from build123d import *

# Parameters (mm, degrees)
Y_KSEKLIK_EKSTR_ZYON1_DEPTH = 5
Y_KSEKLIK_EKSTR_ZYON2_DEPTH = 11.35
Y_KSEKLIK_EKSTR_ZYON3_DEPTH = 2.45
Y_KSEKLIK_EKSTR_ZYON4_DEPTH = 4
IZIM5_R                     = 5.65
Y_KSEKLIK_EKSTR_ZYON5_DEPTH = 4.3
IZIM7_R                     = 0.75
Y_KSEKLIK_EKSTR_ZYON6_DEPTH = 2.9
RADYUS1_R                   = 0.1
IZIM8_R                     = 0.6
Y_KSEKLIK_EKSTR_ZYON7_DEPTH = 3
SKETCH1_OUTSIDE_W           = 23.446
SKETCH1_OUTSIDE_H           = 43.396
SKETCH1_OUTSIDE_W_2         = 11.9
SKETCH1_OUTSIDE_H_2         = 23.420918094
CUT_EXTRUDE1_DEPTH          = 2.45


with BuildPart() as part:
    # Çizim1 → Yükseklik-Ekstrüzyon1 (new body)
    with BuildSketch(Plane(origin=(0, 0, 0), x_dir=(1, 0, 0), z_dir=(0, 1, 0))):
        with BuildLine():
            Line((-5.65, -11.425), (5.65, -11.425))
            ThreePointArc((5.65, -11.425), (6.003553391, -11.278553391), (6.15, -10.925))
            Line((6.15, -10.925), (6.15, 10.925))
            ThreePointArc((6.15, 10.925), (6.003553391, 11.278553391), (5.65, 11.425))
            Line((5.65, 11.425), (-5.65, 11.425))
            ThreePointArc((-5.65, 11.425), (-6.003553391, 11.278553391), (-6.15, 10.925))
            Line((-6.15, 10.925), (-6.15, -10.925))
            ThreePointArc((-6.15, -10.925), (-6.003553391, -11.278553391), (-5.65, -11.425))
        make_face()
    extrude(amount=Y_KSEKLIK_EKSTR_ZYON1_DEPTH)

    # Çizim2 → Yükseklik-Ekstrüzyon2 (add)
    with BuildSketch(Plane(origin=(0, 5, 0), x_dir=(1, 0, 0), z_dir=(0, 1, 0))):
        with BuildLine():
            Line((-5.6, -11.35), (5.6, -11.35))
            ThreePointArc((5.6, -11.35), (5.953553391, -11.203553391), (6.1, -10.85))
            Line((6.1, -10.85), (6.1, 10.85))
            ThreePointArc((6.1, 10.85), (5.953553391, 11.203553391), (5.6, 11.35))
            Line((5.6, 11.35), (-5.6, 11.35))
            ThreePointArc((-5.6, 11.35), (-5.953553391, 11.203553391), (-6.1, 10.85))
            Line((-6.1, 10.85), (-6.1, -10.85))
            ThreePointArc((-6.1, -10.85), (-5.953553391, -11.203553391), (-5.6, -11.35))
        make_face()
    extrude(amount=Y_KSEKLIK_EKSTR_ZYON2_DEPTH)

    # Çizim3 → Yükseklik-Ekstrüzyon3 (add)
    with BuildSketch(Plane(origin=(0, 16.35, 0), x_dir=(1, 0, 0), z_dir=(0, 1, 0))):
        with BuildLine():
            Line((-5.95, 15.625), (-5.95, 11.207071421))
            ThreePointArc((-5.95, 11.207071421), (-5.789029481, 11.31289076), (-5.6, 11.35))
            Line((-5.6, 11.35), (5.6, 11.35))
            ThreePointArc((5.6, 11.35), (5.789029481, 11.31289076), (5.95, 11.207071421))
            Line((5.95, 11.207071421), (5.95, 15.625))
            ThreePointArc((5.95, 15.625), (5.803553391, 15.978553391), (5.45, 16.125))
            Line((5.45, 16.125), (0.5, 16.125))
            Line((0.5, 16.125), (0.5, 14.991025404))
            ThreePointArc((0.5, 14.991025404), (0, 13.125), (-0.5, 14.991025404))
            Line((-0.5, 14.991025404), (-0.5, 16.125))
            Line((-0.5, 16.125), (-5.45, 16.125))
            ThreePointArc((-5.45, 16.125), (-5.803553391, 15.978553391), (-5.95, 15.625))
        make_face()
        with BuildLine():
            Line((-5.95, 11.207071421), (-5.95, -11.207071421))
            ThreePointArc((-5.95, -11.207071421), (-5.789029481, -11.31289076), (-5.6, -11.35))
            Line((-5.6, -11.35), (5.6, -11.35))
            ThreePointArc((5.6, -11.35), (5.789029481, -11.31289076), (5.95, -11.207071421))
            Line((5.95, -11.207071421), (5.95, 11.207071421))
            ThreePointArc((5.95, 11.207071421), (5.789029481, 11.31289076), (5.6, 11.35))
            Line((5.6, 11.35), (-5.6, 11.35))
            ThreePointArc((-5.6, 11.35), (-5.789029481, 11.31289076), (-5.95, 11.207071421))
        make_face()
        with BuildLine():
            ThreePointArc((-5.95, -15.625), (-5.803553391, -15.978553391), (-5.45, -16.125))
            Line((-5.45, -16.125), (-0.5, -16.125))
            Line((-0.5, -16.125), (-0.5, -14.991025404))
            ThreePointArc((-0.5, -14.991025404), (0, -13.125), (0.5, -14.991025404))
            Line((0.5, -14.991025404), (0.5, -16.125))
            Line((0.5, -16.125), (5.45, -16.125))
            ThreePointArc((5.45, -16.125), (5.803553391, -15.978553391), (5.95, -15.625))
            Line((5.95, -15.625), (5.95, -11.207071421))
            ThreePointArc((5.95, -11.207071421), (5.789029481, -11.31289076), (5.6, -11.35))
            Line((5.6, -11.35), (-5.6, -11.35))
            ThreePointArc((-5.6, -11.35), (-5.789029481, -11.31289076), (-5.95, -11.207071421))
            Line((-5.95, -11.207071421), (-5.95, -15.625))
        make_face()
    extrude(amount=Y_KSEKLIK_EKSTR_ZYON3_DEPTH)

    # Çizim4 → Yükseklik-Ekstrüzyon4 (add)
    with BuildSketch(Plane(origin=(0, 18.8, 0), x_dir=(1, 0, 0), z_dir=(0, 1, 0))):
        with BuildLine():
            Line((-5.4, -11.2), (5.4, -11.2))
            ThreePointArc((5.4, -11.2), (5.753553391, -11.053553391), (5.9, -10.7))
            Line((5.9, -10.7), (5.9, 10.7))
            ThreePointArc((5.9, 10.7), (5.753553391, 11.053553391), (5.4, 11.2))
            Line((5.4, 11.2), (-5.4, 11.2))
            ThreePointArc((-5.4, 11.2), (-5.753553391, 11.053553391), (-5.9, 10.7))
            Line((-5.9, 10.7), (-5.9, -10.7))
            ThreePointArc((-5.9, -10.7), (-5.753553391, -11.053553391), (-5.4, -11.2))
        make_face()
    extrude(amount=Y_KSEKLIK_EKSTR_ZYON4_DEPTH)

    # Çizim5 → Yükseklik-Ekstrüzyon5 (add)
    with BuildSketch(Plane(origin=(0, 22.8, 0), x_dir=(1, 0, 0), z_dir=(0, 1, 0))):
        with Locations((0, 5.45)):
            Circle(IZIM5_R)
        with BuildLine():
            ThreePointArc((-2.6, -0.85), (0, -3.45), (2.6, -0.85))
            Line((2.6, -0.85), (2.6, 0.433776321))
            ThreePointArc((2.6, 0.433776321), (0, -0.2), (-2.6, 0.433776321))
            Line((-2.6, 0.433776321), (-2.6, -0.85))
        make_face()
    extrude(amount=Y_KSEKLIK_EKSTR_ZYON5_DEPTH)

    # Çizim7 → Yükseklik-Ekstrüzyon6 (add)
    # profile 1 of 21: a face of its own
    with BuildSketch(Plane(origin=(0, 27.1, 0), x_dir=(1, 0, 0), z_dir=(0, 1, 0))):
        Polygon((1.982489516, 6.460128862), (1.573312588, 7.023312588), (1.010128862, 7.432489516), (0.348066685, 7.647606558), (-0.348066685, 7.647606558), (-1.010128862, 7.432489516), (-1.573312588, 7.023312588), (-1.982489516, 6.460128862), (-2.197606558, 5.798066685), (-2.197606558, 5.101933315), (-1.982489516, 4.439871138), (-1.573312588, 3.876687412), (-1.010128862, 3.467510484), (-0.348066685, 3.252393442), (0.348066685, 3.252393442), (1.010128862, 3.467510484), (1.573312588, 3.876687412), (1.982489516, 4.439871138), (2.197606558, 5.101933315), (2.197606558, 5.798066685), align=None)
        with Locations(Location((0, 5.45, 0), (0, 0, 270))):
            Circle(IZIM7_R, mode=Mode.SUBTRACT)
    # profile 2 of 21: a face of its own
    with BuildSketch(Plane(origin=(0, 27.1, 0), x_dir=(1, 0, 0), z_dir=(0, 1, 0))):
        Polygon((-0.749366211, 7.756312052), (-0.348066685, 7.647606558), (-1.010128862, 7.432489516), align=None)
    # profile 3 of 21: a face of its own
    with BuildSketch(Plane(origin=(0, 27.1, 0), x_dir=(1, 0, 0), z_dir=(0, 1, 0))):
        Polygon((0, 7.875), (0.348066685, 7.647606558), (-0.348066685, 7.647606558), align=None)
    # profile 4 of 21: a face of its own
    with BuildSketch(Plane(origin=(0, 27.1, 0), x_dir=(1, 0, 0), z_dir=(0, 1, 0))):
        Polygon((-1.425379237, 7.411866211), (-1.010128862, 7.432489516), (-1.573312588, 7.023312588), align=None)
    # profile 5 of 21: a face of its own
    with BuildSketch(Plane(origin=(0, 27.1, 0), x_dir=(1, 0, 0), z_dir=(0, 1, 0))):
        Polygon((-1.961866211, 6.875379237), (-1.573312588, 7.023312588), (-1.982489516, 6.460128862), align=None)
    # profile 6 of 21: a face of its own
    with BuildSketch(Plane(origin=(0, 27.1, 0), x_dir=(1, 0, 0), z_dir=(0, 1, 0))):
        Polygon((-2.306312052, 6.199366211), (-1.982489516, 6.460128862), (-2.197606558, 5.798066685), align=None)
    # profile 7 of 21: a face of its own
    with BuildSketch(Plane(origin=(0, 27.1, 0), x_dir=(1, 0, 0), z_dir=(0, 1, 0))):
        Polygon((-2.306312052, 4.700633789), (-2.197606558, 5.101933315), (-1.982489516, 4.439871138), align=None)
    # profile 8 of 21: a face of its own
    with BuildSketch(Plane(origin=(0, 27.1, 0), x_dir=(1, 0, 0), z_dir=(0, 1, 0))):
        Polygon((-2.425, 5.45), (-2.197606558, 5.798066685), (-2.197606558, 5.101933315), align=None)
    # profile 9 of 21: a face of its own
    with BuildSketch(Plane(origin=(0, 27.1, 0), x_dir=(1, 0, 0), z_dir=(0, 1, 0))):
        Polygon((-1.961866211, 4.024620763), (-1.982489516, 4.439871138), (-1.573312588, 3.876687412), align=None)
    # profile 10 of 21: a face of its own
    with BuildSketch(Plane(origin=(0, 27.1, 0), x_dir=(1, 0, 0), z_dir=(0, 1, 0))):
        Polygon((-1.425379237, 3.488133789), (-1.573312588, 3.876687412), (-1.010128862, 3.467510484), align=None)
    # profile 11 of 21: a face of its own
    with BuildSketch(Plane(origin=(0, 27.1, 0), x_dir=(1, 0, 0), z_dir=(0, 1, 0))):
        Polygon((-0.749366211, 3.143687948), (-1.010128862, 3.467510484), (-0.348066685, 3.252393442), align=None)
    # profile 12 of 21: a face of its own
    with BuildSketch(Plane(origin=(0, 27.1, 0), x_dir=(1, 0, 0), z_dir=(0, 1, 0))):
        Polygon((0, 3.025), (-0.348066685, 3.252393442), (0.348066685, 3.252393442), align=None)
    # profile 13 of 21: a face of its own
    with BuildSketch(Plane(origin=(0, 27.1, 0), x_dir=(1, 0, 0), z_dir=(0, 1, 0))):
        Polygon((0.749366211, 3.143687948), (0.348066685, 3.252393442), (1.010128862, 3.467510484), align=None)
    # profile 14 of 21: a face of its own
    with BuildSketch(Plane(origin=(0, 27.1, 0), x_dir=(1, 0, 0), z_dir=(0, 1, 0))):
        Polygon((0.749366211, 7.756312052), (1.010128862, 7.432489516), (0.348066685, 7.647606558), align=None)
    # profile 15 of 21: a face of its own
    with BuildSketch(Plane(origin=(0, 27.1, 0), x_dir=(1, 0, 0), z_dir=(0, 1, 0))):
        Polygon((1.425379237, 7.411866211), (1.573312588, 7.023312588), (1.010128862, 7.432489516), align=None)
    # profile 16 of 21: a face of its own
    with BuildSketch(Plane(origin=(0, 27.1, 0), x_dir=(1, 0, 0), z_dir=(0, 1, 0))):
        Polygon((1.961866211, 6.875379237), (1.982489516, 6.460128862), (1.573312588, 7.023312588), align=None)
    # profile 17 of 21: a face of its own
    with BuildSketch(Plane(origin=(0, 27.1, 0), x_dir=(1, 0, 0), z_dir=(0, 1, 0))):
        Polygon((2.306312052, 6.199366211), (2.197606558, 5.798066685), (1.982489516, 6.460128862), align=None)
    # profile 18 of 21: a face of its own
    with BuildSketch(Plane(origin=(0, 27.1, 0), x_dir=(1, 0, 0), z_dir=(0, 1, 0))):
        Polygon((2.425, 5.45), (2.197606558, 5.101933315), (2.197606558, 5.798066685), align=None)
    # profile 19 of 21: a face of its own
    with BuildSketch(Plane(origin=(0, 27.1, 0), x_dir=(1, 0, 0), z_dir=(0, 1, 0))):
        Polygon((2.306312052, 4.700633789), (1.982489516, 4.439871138), (2.197606558, 5.101933315), align=None)
    # profile 20 of 21: a face of its own
    with BuildSketch(Plane(origin=(0, 27.1, 0), x_dir=(1, 0, 0), z_dir=(0, 1, 0))):
        Polygon((1.961866211, 4.024620763), (1.573312588, 3.876687412), (1.982489516, 4.439871138), align=None)
    # profile 21 of 21: a face of its own
    with BuildSketch(Plane(origin=(0, 27.1, 0), x_dir=(1, 0, 0), z_dir=(0, 1, 0))):
        Polygon((1.425379237, 3.488133789), (1.010128862, 3.467510484), (1.573312588, 3.876687412), align=None)
    extrude(amount=Y_KSEKLIK_EKSTR_ZYON6_DEPTH)

    # Radyus1
    radyus1_edges = [part.edges().sort_by_distance(p)[0] for p in [
        (0, 22.8, -11.2),
        (-5.753553391, 22.8, -11.053553391),
        (-5.9, 22.8, 0),
        (-5.753553391, 22.8, 11.053553391),
        (0, 0, 11.425),
        (0, 22.8, 11.2),
        (-6.003553391, 0, 11.278553391),
        (-6.15, 0, 0),
        (-6.003553391, 0, -11.278553391),
        (0, 0, -11.425),
        (6.003553391, 0, -11.278553391),
        (6.15, 0, 0),
        (6.003553391, 0, 11.278553391),
        (5.753553391, 22.8, 11.053553391),
        (5.9, 22.8, 0),
        (5.753553391, 22.8, -11.053553391),
    ]]
    fillet(radyus1_edges, radius=RADYUS1_R - 0.0001)  # a hair under: the kernel refuses the full size

    # Çizim8 → Yükseklik-Ekstrüzyon7 (add)
    with BuildSketch(Plane(origin=(0, 0, -11.425), x_dir=(-1, 0, 0), z_dir=(0, 0, -1))):
        with Locations(Location((-1.25, 4.4, 0), (0, 0, 90))):
            Circle(IZIM8_R)
        with Locations(Location((0, 4.4, 0), (0, 0, 90))):
            Circle(IZIM8_R)
        with Locations(Location((1.25, 4.4, 0), (0, 0, 90))):
            Circle(IZIM8_R)
    extrude(amount=Y_KSEKLIK_EKSTR_ZYON7_DEPTH)

    # Sketch1 outside → Cut-Extrude1 (cut)
    with BuildSketch(Plane(origin=(0, 18.8, 0), x_dir=(1, 0, 0), z_dir=(0, 1, 0))):
        Rectangle(SKETCH1_OUTSIDE_W, SKETCH1_OUTSIDE_H)
        with Locations((0, -0.105309884)):
            Rectangle(SKETCH1_OUTSIDE_W_2, SKETCH1_OUTSIDE_H_2, mode=Mode.SUBTRACT)
    extrude(amount=-CUT_EXTRUDE1_DEPTH, mode=Mode.SUBTRACT)


solid = part.part
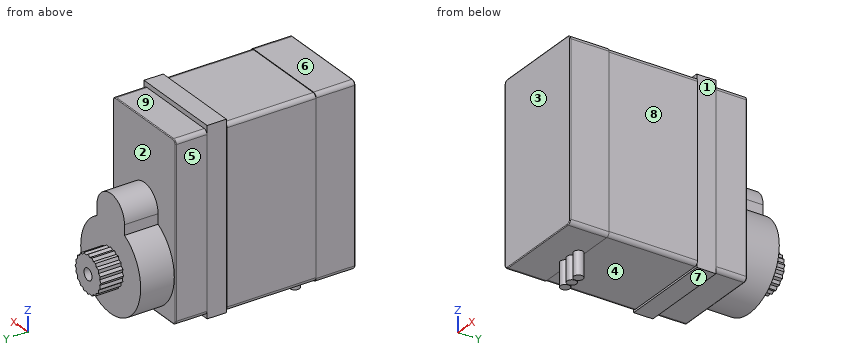
Geometry: final body of the model. Coordinates: model frame, mm. Face numbers are marked on the shaded views. A direction names the side the tool comes from. Round coordinates to 2 decimals unless told otherwise and drop trailing zeros. Write each loop counter-clockwise with the first axis right and the second up, starting at its lowest first coordinate (ties: lowest second). Pieces come first, ordered by that corner, then holes. Notation, with made-up numbers: M 64,79.5 L 100,79.5 A31 cw 100,116.5 Z; hole C 76.5,40.5 d10. An arc over 180 degrees is marked long. Write item = value, one per line.
Item 1: Section query C-C on x = -4. Return loops of the section in (y, z) (3 decimals), then the cut area to 3 significant figures.
Findings:
outline = M 0,-11.325 A0.1 ccw 0.1,-11.425 L 5,-11.425 L 5,-11.35 L 16.35,-11.35 L 16.35,-11.605 L 18.8,-11.605 L 18.8,-11.2 L 22.7,-11.2 A0.1 ccw 22.8,-11.1 L 22.8,-9.44 L 27.1,-9.44 L 27.1,-1.46 L 22.8,-1.46 L 22.8,11.1 A0.1 ccw 22.7,11.2 L 18.8,11.2 L 18.8,11.816 L 16.35,11.816 L 16.35,11.35 L 5,11.35 L 5,11.425 L 0.1,11.425 A0.1 ccw 0,11.325 Z
area = 553 mm^2
Item 2: Access query for the marked faces 5, 6, 7, 8 and 9. Directions: +Z, -Z, +X, -X, +Y, -Y. A direction counts if a zero-diameter tool reaches every point of the face in a straight line with its end or side. Return the directions, or none.
Findings:
face_5 = +Z, -Z, -X, +Y
face_6 = +Z, +X, -X, -Y
face_7 = -Z, +X, -X, +Y
face_8 = +Z, -Z, +X, +Y
face_9 = +Z, +X, -X, +Y
Item 3: Pull-direction query (Y, two-part tool) for the marked faces 1, 2, 3 and 4; classes: pulls with the +Y half, pulls with the -Y half, needs draft (parallel to the pull), parting line crosses it, or undercut.
Findings:
face_1 = needs draft
face_2 = pulls with the +Y half
face_3 = pulls with the -Y half
face_4 = undercut
Item 4: Material intervals for line 1 along Y through (x, z) = (-3.25, -8.75); line 2 along Y through (x, z) = (5.5, -1.5); line 3 along X through (y, z) = (21.25, -3.5), sorted ascending. Write a range as [from, to].
Findings:
line_1 = [0, 27.1]
line_2 = [0, 22.8]
line_3 = [-5.9, 5.9]
Item 5: Section query A-A on y = 14.5. Return loops of the section in (x, z), then the cut area to 3 significant figures.
Findings:
outline = M -6.1,-10.85 A0.5 ccw -5.6,-11.35 L 5.6,-11.35 A0.5 ccw 6.1,-10.85 L 6.1,10.85 A0.5 ccw 5.6,11.35 L -5.6,11.35 A0.5 ccw -6.1,10.85 Z
area = 277 mm^2
Item 6: Section query B-B on z = 0. Return loops of the section in (x, y).
Findings:
outline = M -6.15,0.1 A0.1 ccw -6.05,0 L 6.05,0 A0.1 ccw 6.15,0.1 L 6.15,5 L 6.1,5 L 6.1,16.35 L 5.95,16.35 L 5.95,18.8 L 5.9,18.8 L 5.9,22.7 A0.1 ccw 5.8,22.8 L 2.6,22.8 L 2.6,27.1 L -2.6,27.1 L -2.6,22.8 L -5.8,22.8 A0.1 ccw -5.9,22.7 L -5.9,18.8 L -5.95,18.8 L -5.95,16.35 L -6.1,16.35 L -6.1,5 L -6.15,5 Z
Item 7: Pin query (flat end, axial travel): P1, Ø1.5, axis at x = 2, y = 2, coming from the -Z side (3 decimals); P2, Ø1, axis at y = 16.5, z = -11, coming from the -X side; P3, Ø1.5, axis at x = -2.5, z = -8, coming from the +Y side. Return the tip coordinate at first contact, or that it passes through.
Findings:
P1 = -11.425
P2 = -6.1
P3 = 27.1
Item 8: Section query D-D on y = 4.4. Return loops of the section in (x, z) (3 decimals), then the cut area to 3 significant figures.
Findings:
outline = M -6.15,-10.925 A0.5 ccw -5.65,-11.425 L -1.85,-11.425 L -1.85,-14.425 L -0.65,-14.425 L -0.65,-11.425 L -0.6,-11.425 L -0.6,-14.425 L 0.6,-14.425 L 0.6,-11.425 L 0.65,-11.425 L 0.65,-14.425 L 1.85,-14.425 L 1.85,-11.425 L 5.65,-11.425 A0.5 ccw 6.15,-10.925 L 6.15,10.925 A0.5 ccw 5.65,11.425 L -5.65,11.425 A0.5 ccw -6.15,10.925 Z
area = 292 mm^2
